CAD build for the part. Positions are in the model's coordinates, mm. A direction names the side the tool comes from. Give positions to 0.01 mm unless a question says otherwise; leave off trailing zeros. Order: outer loops, then holes, each group sorted by start corner. A loop starts at its lowest first (then second) coordinate and runs counter-clockwise, first axis right, second up.
Item 1: Band-saw the part on A-A on y = 50. Give the cut face in (x, z), plus the area to 3 significant figures.
Item 2: Which spindle directions (+Z, -Z, +X, -X, +Y, -Y) get a long thin tool onto all of the face, cutting with end or side? Do faces 4 (the flat face through (80, 39, 128)), 5 (the cylindrical face through (38.041, 57.892, 7.605)). Say none if no direction does.
Item 3: Flat gauge pin, fed straight in: P1, Ø4, axis at x = 50, z = 85.5, coming from the -Y side. Where does the tip first touch, or does it go through?
Item 4: Wall check: L1, parallel to X at y = 60, z = 10.5 (3 decimals); L2, parallel to Z at x = 39.5, y = 63; L3, parallel to Z at x = 46.5, y = 39. Give the ranges that are in metal, low to high.
Item 5: Two-plate mould, pull along Z, no slides. Class faces 1 (the flat face through (0, 39, 128)), 2 (the cylindrical face through (41.632, 30.42, 207.435)), 3 (the conical face through (39.79, 60.17, 16.24)): released by +Z, released by -Z, zero draft, split by the parting line, or undercut.
```python
from build123d import *

# Parameters (mm, degrees)
F0_W     = 80
F0_H     = 80
F1_DEPTH = 260
F3_D     = 25
F3_DEPTH = 60
F3_TIP   = 7.5107577378
F5_D     = 5
F5_DEPTH = 15
F5_TIP   = 1.5021515476


with BuildPart() as f1:
    # F0 (on Top) → F1 (new body)
    with BuildSketch(Plane.XY):
        with Locations((40, 40)):
            Rectangle(F0_W, F0_H)
    extrude(amount=F1_DEPTH)

    # F3
    with Locations(Plane.XZ):
        with Locations((40.004914752, 195.0411053359)):
            Hole(F3_D / 2, depth=F3_DEPTH)
            with Locations((0, 0, -(F3_DEPTH + F3_TIP / 2))):  # 118° drill point
                Cone(0, F3_D / 2, F3_TIP, mode=Mode.SUBTRACT)

    # F5
    with Locations(Plane(origin=(0, 0, 0), x_dir=(1, 0, 0), z_dir=(0, 0, -1))):
        with Locations((39.3849909306, -20), (39.3849909306, -60)):
            Hole(F5_D / 2, depth=F5_DEPTH)
            with Locations((0, 0, -(F5_DEPTH + F5_TIP / 2))):  # 118° drill point
                Cone(0, F5_D / 2, F5_TIP, mode=Mode.SUBTRACT)


solid = f1.part
```
The answers:
1. outline: (0, 0) - (80, 0) - (80, 260) - (0, 260) - close; hole circle Ø25 at (40, 195.04)
1. area: 20,300 mm2
2. face 4: +Z, -Z, +X, +Y, -Y
2. face 5: -Z
3. P1: stops at y = 0
4. L1: x = 0 to 36.885, 41.885 to 80
4. L2: z = 0 to 187.55, 202.53 to 260
4. L3: z = 0 to 184.36, 205.72 to 260
5. face 1: zero draft
5. face 2: undercut
5. face 3: released by -Z
